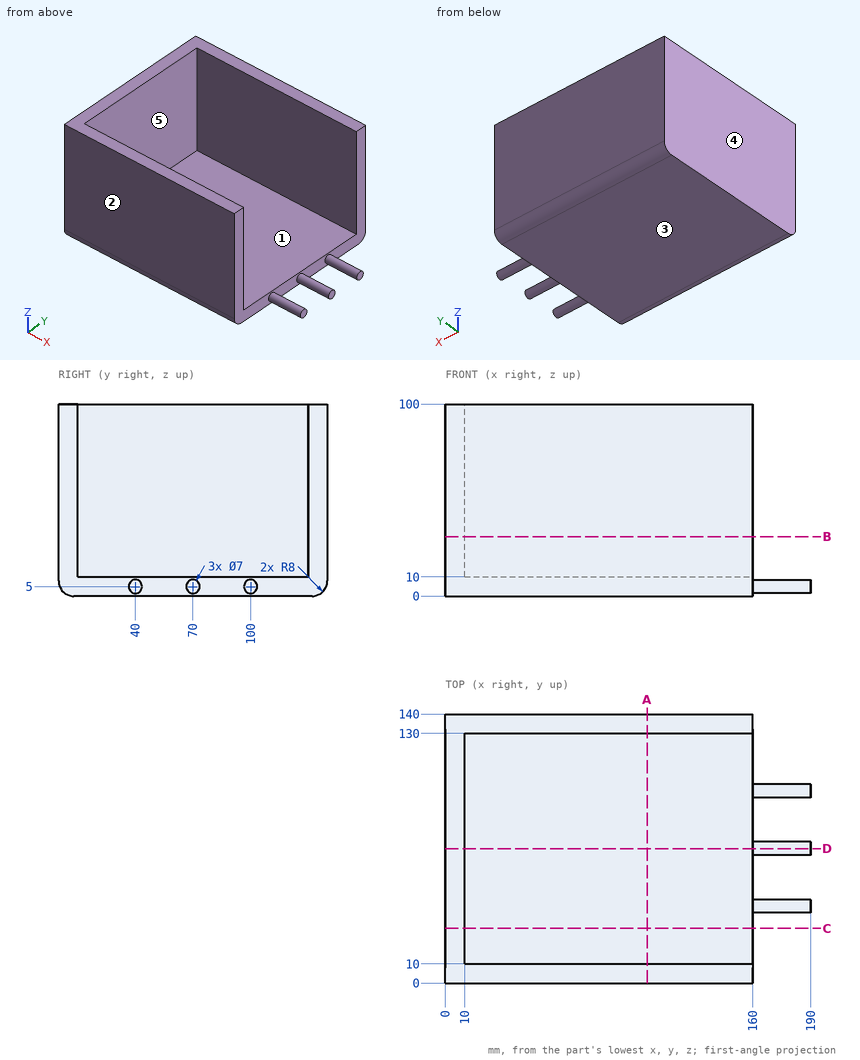
Source: three-view drawing plus pictorial views. Frame: mm from the lowest corner of the part. A direction names the side the tool comes from. Coordinates: 2 decimals unless noted, no trailing zeros. Order: outer loops, then holes, each group sorted by start corner. A loop starts at its lowest first (then second) coordinate and runs counter-clockwise, first axis right, second up. Notation, with made-up numbers: (-14, 70.25) -> (13, 70.25) arc R22 ccw to (13, 78.25) -> close; hole circle Ø9 at (76, 38.25). An arc over 180 degrees is marked (long way). Write item = value, one per line.
(1) Pull-direction query (Y, two-part tool) for the marked faces 1, 2 and 3; classes: pulls with the +Y half, pulls with the -Y half, needs draft (parallel to the pull), parting line crosses it, or undercut.
Solved:
face_1 = undercut
face_2 = pulls with the -Y half
face_3 = needs draft
(2) Cut plane A-A on x = 105. Return loops of the section in (y, z), plus the area to 3 significant figures.
Solved:
outline = (0, 8) arc R8 ccw to (8, 0) -> (132, 0) arc R8 ccw to (140, 8) -> (140, 100) -> (130, 100) -> (130, 10) -> (10, 10) -> (10, 100) -> (0, 100) -> close
area = 3,170 mm²
(3) Pin query (flat end, axial travel): pin 1 Ø3 at (y, z) = (54.5, 49) entering from -X; pin 2 Ø4 at (x, y) = (92.5, 95) entering from +Z; pin 3 Ø1 at (y, z) = (28.5, 84.5) entering from +X. Return the tip coordinate at first contact, or that it passes through.
Solved:
pin_1 = 0
pin_2 = 10
pin_3 = 10
(4) Line query: line 1 (Y direction, x = 36, z = 48); line 2 (Z direction, x = 87, y = 109). Output: solid intervals per line, ascending.
Solved:
line_1 = 0 to 10, 130 to 140
line_2 = 0 to 10
(5) Access query for the marked faces 4 and 5. Directions: +Z, -Z, +X, -X, +Y, -Y. A direction counts if a zero-diameter tool reaches every point of the face in a straight line with its end or side. Return the directions, or none.
Solved:
face_4 = +Z, -Z, -X, +Y, -Y
face_5 = +Z, +X
(6) Cut plane C-C on y = 28.5. Return loops of the section in (x, z), plus the area to 3 significant figures.
Solved:
outline = (0, 0) -> (160, 0) -> (160, 10) -> (10, 10) -> (10, 100) -> (0, 100) -> close
area = 2,500 mm²
(7) Cut plane B-B on z = 31. Return loops of the section in (x, y).
Solved:
outline = (0, 0) -> (160, 0) -> (160, 10) -> (10, 10) -> (10, 130) -> (160, 130) -> (160, 140) -> (0, 140) -> close
(8) Cut plane D-D on y = 70. Return loops of the section in (x, z).
Solved:
outline = (0, 0) -> (160, 0) -> (160, 1.5) -> (190, 1.5) -> (190, 8.5) -> (160, 8.5) -> (160, 10) -> (10, 10) -> (10, 100) -> (0, 100) -> close
